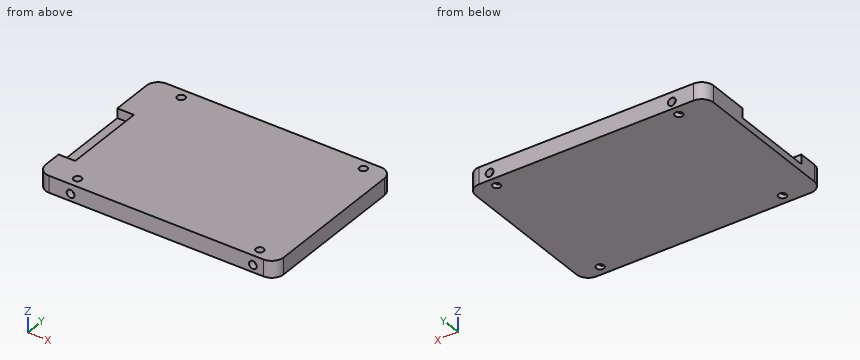
```python
from build123d import *

# Parameters (mm, degrees)
F0_W           = 100
F0_H           = 70
F1_DEPTH       = 7
F2_R           = 5
F6_D           = 3.3
F6_DEPTH       = 7
F6_TIP         = 0.9914200214
F6_ON_F5_D     = 3.3
F6_ON_F5_DEPTH = 7
F6_ON_F5_TIP   = 0.9914200214
F6_ON_F4_D     = 3.3
F6_ON_F4_DEPTH = 7
F6_ON_F4_TIP   = 0.9914200214
F7_W           = 7
F7_H           = 35
F8_DEPTH       = 4


with BuildPart() as f1:
    # F0 (on Top) → F1 (new body)
    with BuildSketch(Plane.XY):
        Rectangle(F0_W, F0_H)
    extrude(amount=F1_DEPTH)

    # F2
    f2_edges = [f1.edges().sort_by_distance(p)[0] for p in [
        (-50, -35, 3.5),
        (50, -35, 3.5),
        (-50, 35, 3.5),
        (50, 35, 3.5),
    ]]
    fillet(f2_edges, radius=F2_R)

    # F6
    with Locations(Plane.XY.offset(7)):
        with Locations((-36, 30.855), (-36, -30.855), (40.6, -30.855), (40.6, 30.855)):
            Hole(F6_D / 2, depth=F6_DEPTH)
            with Locations((0, 0, -(F6_DEPTH + F6_TIP / 2))):  # 118° drill point
                Cone(0, F6_D / 2, F6_TIP, mode=Mode.SUBTRACT)

    # F6 on F5
    with Locations(Plane(origin=(0, 35, 0), x_dir=(-1, 0, 0), z_dir=(0, 1, 0))):
        with Locations((-40.6, 3), (36, 3)):
            Hole(F6_ON_F5_D / 2, depth=F6_ON_F5_DEPTH)
            with Locations((0, 0, -(F6_ON_F5_DEPTH + F6_ON_F5_TIP / 2))):  # 118° drill point
                Cone(0, F6_ON_F5_D / 2, F6_ON_F5_TIP, mode=Mode.SUBTRACT)

    # F6 on F4
    with Locations(Plane.XZ.offset(35)):
        with Locations((-36, 3), (40.6, 3)):
            Hole(F6_ON_F4_D / 2, depth=F6_ON_F4_DEPTH)
            with Locations((0, 0, -(F6_ON_F4_DEPTH + F6_ON_F4_TIP / 2))):  # 118° drill point
                Cone(0, F6_ON_F4_D / 2, F6_ON_F4_TIP, mode=Mode.SUBTRACT)

    # F7 (on face) → F8 (cut)
    with BuildSketch(Plane.XY.offset(7)):
        with Locations((-46.5, -4.8)):
            Rectangle(F7_W, F7_H)
    extrude(amount=-F8_DEPTH, mode=Mode.SUBTRACT)


solid = f1.part
```
Input: part model. Units: mm. Frame: model coordinates. Coordinates: 2 decimals unless noted, no trailing zeros. Loops run counter-clockwise (first coordinate to the right, second up) from the corner with the lowest first, then second, coordinate; pieces in that order, holes last. Notation, with made-up numbers: (-39.75, -4) -> (3.25, -4) arc R23 ccw to (3.25, 10) -> close; hole circle Ø11 at (16, 47). An arc over 180 degrees is marked (long way). Use a Markdown table: item, result.
1) Contact query for flat-ended pins moving along their axis: pin 1 (3 mm diameter, centred on x = -36, z = 3, fed in from -Y); pin 2 (2 mm diameter, centred on x = 40.6, z = 3, fed in from +Y); pin 3 (2 mm diameter, centred on y = -2, z = 5, fed in from -X); pin 4 (5.5 mm diameter, centred on x = 40.6, y = -30.855, fed in from -Z). Output: stop coordinate, or through.
Results found:
| item | result |
|---|---|
| pin 1 | stops at y = -27.91 |
| pin 2 | stops at y = 27.61 |
| pin 3 | stops at x = -43 |
| pin 4 | stops at z = 0 |
2) Cut plane B-B (y = -13). Return the cut outline in (x, z).
Results found:
| item | result |
|---|---|
| outline | (-50, 0) -> (50, 0) -> (50, 7) -> (-43, 7) -> (-43, 3) -> (-50, 3) -> close |
3) Cut plane A-A (z = 5.75). Return the cut outline in (x, y) (3 decimals).
Results found:
| item | result |
|---|---|
| outline | (-50, -30) arc R5 ccw to (-45, -35) -> (45, -35) arc R5 ccw to (50, -30) -> (50, 30) arc R5 ccw to (45, 35) -> (-45, 35) arc R5 ccw to (-50, 30) -> (-50, 12.7) -> (-43, 12.7) -> (-43, -22.3) -> (-50, -22.3) -> close; hole circle Ø3.3 at (-36, -30.855); hole circle Ø3.3 at (-36, 30.855); hole circle Ø3.3 at (40.6, -30.855); hole circle Ø3.3 at (40.6, 30.855) |
4) Material intervals for line 1 along X through (y, z) = (-29, 2.75); line 2 along Y through (x, z) = (40.6, 0.9) (3 decimals); line 3 along X through (y, z) = (-32.8, 3), sorted ascending. Write a range as from..to.
Results found:
| item | result |
|---|---|
| line 1 | x = -50..-37.63, -34.37..38.97, 42.23..50 |
| line 2 | y = -35..-32.505, -29.205..29.205, 32.505..35 |
| line 3 | x = -49.14..-37.65, -34.35..38.95, 42.25..49.14 |
